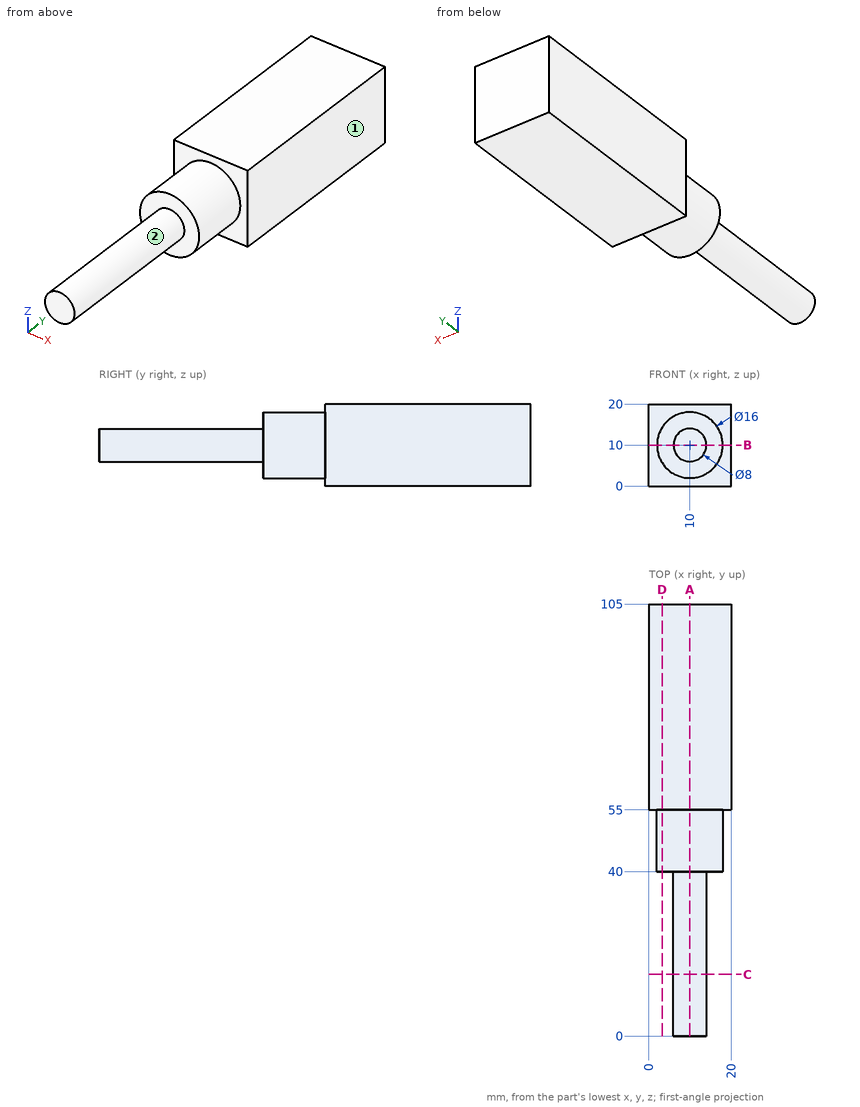
Geometry: see drawing. Coordinates: mm, zero at the bounding-box minimum. A direction names the side the tool comes from. Coordinates: 2 decimals unless noted, no trailing zeros. Write each loop counter-clockwise with the first axis right and the second up, starting at its lowest first coordinate (ties: lowest second). Pieces come first, ordered by that corner, then holes.
1) Set-up query: the marked faces 1 and 2. Return all of +Z, -Z, +X, -X, +Y, -Y with unobstructed straight access to the full face (end or side cutting, diameter ignored); none if empty.
2) Section B-B on z = 10. Output: boundary loops of the cut face in (x, y).
3) Section A-A on x = 10. Output: boundary loops of the cut face in (y, z).
4) Pin query (flat end, axial travel): pin 1 Ø1.5 at (y, z) = (13.5, 10) entering from +X; pin 2 Ø2 at (y, z) = (21, 9) entering from -X; pin 3 Ø5 at (y, z) = (38, 16) entering from +X. Return the tip coordinate at first contact, or that it passes through.
5) Material intervals for line 1 along Y through (x, z) = (14.5, 1.75); line 2 along Y through (x, z) = (15.25, 13.5); line 3 along X through (y, z) = (52, 10.5), sorted ascending.
6) Section C-C on y = 15. Output: boundary loops of the cut face in (x, z).
7) Section D-D on x = 3.25. Output: boundary loops of the cut face in (y, z).
Check result:
1. face 1: +Z, -Z, +X, +Y, -Y
1. face 2: -Y
2. outline: (0, 55) - (2, 55) - (2, 40) - (6, 40) - (6, 0) - (14, 0) - (14, 40) - (18, 40) - (18, 55) - (20, 55) - (20, 105) - (0, 105) - close
3. outline: (0, 6) - (40, 6) - (40, 2) - (55, 2) - (55, 0) - (105, 0) - (105, 20) - (55, 20) - (55, 18) - (40, 18) - (40, 14) - (0, 14) - close
4. pin 1: stops at x = 14
4. pin 2: stops at x = 6
4. pin 3: stops at x = 16.61
5. line 1: y = 55 to 105
5. line 2: y = 40 to 105
5. line 3: x = 2.02 to 17.98
6. outline: circle Ø8 at (10, 10)
7. outline: (40, 5.71) - (55, 5.71) - (55, 0) - (105, 0) - (105, 20) - (55, 20) - (55, 14.29) - (40, 14.29) - close
